Build history of the part. All positions in model axes, mm. A direction names the side the tool comes from. Round coordinates to 2 decimals unless told otherwise and drop trailing zeros. Order: outer loops, then holes, each group sorted by start corner. A loop starts at its lowest first (then second) coordinate and runs counter-clockwise, first axis right, second up. Notation, with made-up numbers: (-38.75, -10) -> (-2.75, -10) arc R4 ccw to (-2.75, -6) -> close; hole circle Ø9 at (24.25, -14.5). An arc over 180 degrees is marked (long way). Use a Markdown table: item, result. Add a question column.
Item 1: Slice it at D-D, the plane x = 55. Give the cut face in (y, z).
Item 2: Slice it at B-B, the plane z = 0. Give the cut face in (x, y).
Item 3: Slice it at A-A, the plane x = -55. Give the cut face in (y, z).
Item 4: Probe L1, parallel to X at y = 4.2, z = 0; L2, parallel to X at y = 0.9, z = 1; L3, parallel to X at y = 5.75, z = -1.5. List the from-to ranges inside material, lowest first.
Item 5: Pin check, flat tips, straight feed: pin 1 (8 mm diameter, centred on x = -18.5, z = -1, fed in from +Y); pin 2 (3 mm diameter, centred on x = -25.5, y = 2, fed in from +Z); pin 3 (1.5 mm diameter, centred on y = 1.5, z = -11, fed in from +X). Stop position of each tip, or through.
Item 6: Two-plate mould, pull along X, no slides. Class faces 4 (the face through (51.095, 4.986, -0.867)), 5 (the face through (53, 6, 2)): released by +X, released by -X, zero draft, split by the parting line, or undercut.
Item 7: Slice it at C-C, the plane y = 2.2. Give the cut face in (x, z), plus the area to 3 significant figures.
Item 8: 3-axis set-ups, long thin cutter, end or side, ignore diameter. For faces 1 (the face through (-40.97, 2.03, -8.26)), 2 (the face through (-58.905, 4.986, -0.867)), 3 (the face through (35.256, 2.028, 8.633)): which of +Z, -Z, +X, -X, +Y, -Y reach the whole face in a straight line?
from build123d import *

# Parameters (mm, degrees)
SKETCH1_R           = 2.1
BOSS_EXTRUDE1_DEPTH = 4
FILLET1_R           = 10
SKETCH2_R           = 4
SKETCH2_R_2         = 2.1
BOSS_EXTRUDE2_DEPTH = 2


with BuildPart() as part:
    # Sketch1 → Boss-Extrude1 (new body)
    with BuildSketch(Plane(origin=(0, 0, 0), x_dir=(1, 0, 0), z_dir=(0, 1, 0))):
        with BuildLine():
            Line((-42.009618943, 7.5), (36.459503782, 7.5))
            ThreePointArc((36.459503782, 7.5), (75, 0), (36.459503782, -7.5))
            Line((36.459503782, -7.5), (-42.009618943, -7.5))
            ThreePointArc((-42.009618943, -7.5), (-70, 0), (-42.009618943, 7.5))
        make_face()
        with Locations(Location((-55, 0, 0), (0, 0, 270))):
            Circle(SKETCH1_R, mode=Mode.SUBTRACT)
        with Locations(Location((55, 0, 0), (0, 0, 270))):
            Circle(SKETCH1_R, mode=Mode.SUBTRACT)
    extrude(amount=BOSS_EXTRUDE1_DEPTH)

    # Fillet1
    fillet1_edges = [part.edges().sort_by_distance(p)[0] for p in [
        (36.459503782, 2, 7.5),
        (-42.009618943, 2, 7.5),
        (-42.009618943, 2, -7.5),
        (36.459503782, 2, -7.5),
    ]]
    fillet(fillet1_edges, radius=FILLET1_R)

    # Sketch2 → Boss-Extrude2 (add)
    # profile 1 of 2: a face of its own
    with BuildSketch(Plane(origin=(0, 4, 0), x_dir=(1, 0, 0), z_dir=(0, 1, 0))):
        with Locations(Location((55, 0, 0), (0, 0, 270))):
            Circle(SKETCH2_R)
        with Locations(Location((55, 0, 0), (0, 0, 270))):
            Circle(SKETCH2_R_2, mode=Mode.SUBTRACT)
    # profile 2 of 2: a face of its own
    with BuildSketch(Plane(origin=(0, 4, 0), x_dir=(1, 0, 0), z_dir=(0, 1, 0))):
        with Locations(Location((-55, 0, 0), (0, 0, 270))):
            Circle(SKETCH2_R)
        with Locations(Location((-55, 0, 0), (0, 0, 270))):
            Circle(SKETCH2_R_2, mode=Mode.SUBTRACT)
    extrude(amount=BOSS_EXTRUDE2_DEPTH)


solid = part.part
Check sheet entries:
| question | item | result |
|---|---|---|
| 1 | outline | (0, -20) -> (4, -20) -> (4, -4) -> (6, -4) -> (6, -2.1) -> (0, -2.1) -> close; (0, 2.1) -> (6, 2.1) -> (6, 4) -> (4, 4) -> (4, 20) -> (0, 20) -> close |
| 2 | outline | (-70, 0) -> (-57.1, 0) -> (-57.1, 6) -> (-59, 6) -> (-59, 4) -> (-70, 4) -> close; (-52.9, 0) -> (52.9, 0) -> (52.9, 6) -> (51, 6) -> (51, 4) -> (-51, 4) -> (-51, 6) -> (-52.9, 6) -> close; (57.1, 0) -> (75, 0) -> (75, 4) -> (59, 4) -> (59, 6) -> (57.1, 6) -> close |
| 3 | outline | (0, -15) -> (4, -15) -> (4, -4) -> (6, -4) -> (6, -2.1) -> (0, -2.1) -> close; (0, 2.1) -> (6, 2.1) -> (6, 4) -> (4, 4) -> (4, 15) -> (0, 15) -> close |
| 4 | L1 | -59 to -57.1, -52.9 to -51, 51 to 52.9, 57.1 to 59 |
| 4 | L2 | -69.97 to -56.85, -53.15 to 53.15, 56.85 to 74.97 |
| 4 | L3 | -58.71 to -56.47, -53.53 to -51.29, 51.29 to 53.53, 56.47 to 58.71 |
| 5 | pin 1 | y = 4 |
| 5 | pin 2 | z = 7.5 |
| 5 | pin 3 | x = 72.17 |
| 6 | face 4 | undercut |
| 6 | face 5 | zero draft |
| 7 | outline | (-44.29, -10.5) arc R10 cw to (-37.15, -7.5) -> (30.63, -7.5) arc R10 cw to (38.76, -11.67) arc R20 ccw (long way) to (38.76, 11.67) arc R10 cw to (30.63, 7.5) -> (-37.15, 7.5) arc R10 cw to (-44.29, 10.5) arc R15 ccw (long way) to start; hole circle Ø4.2 at (-55, 0); hole circle Ø4.2 at (55, 0) |
| 7 | area | 3,090 mm2 |
| 8 | face 1 | -Z, +Y, -Y |
| 8 | face 2 | +Y |
| 8 | face 3 | +Z, +Y, -Y |
